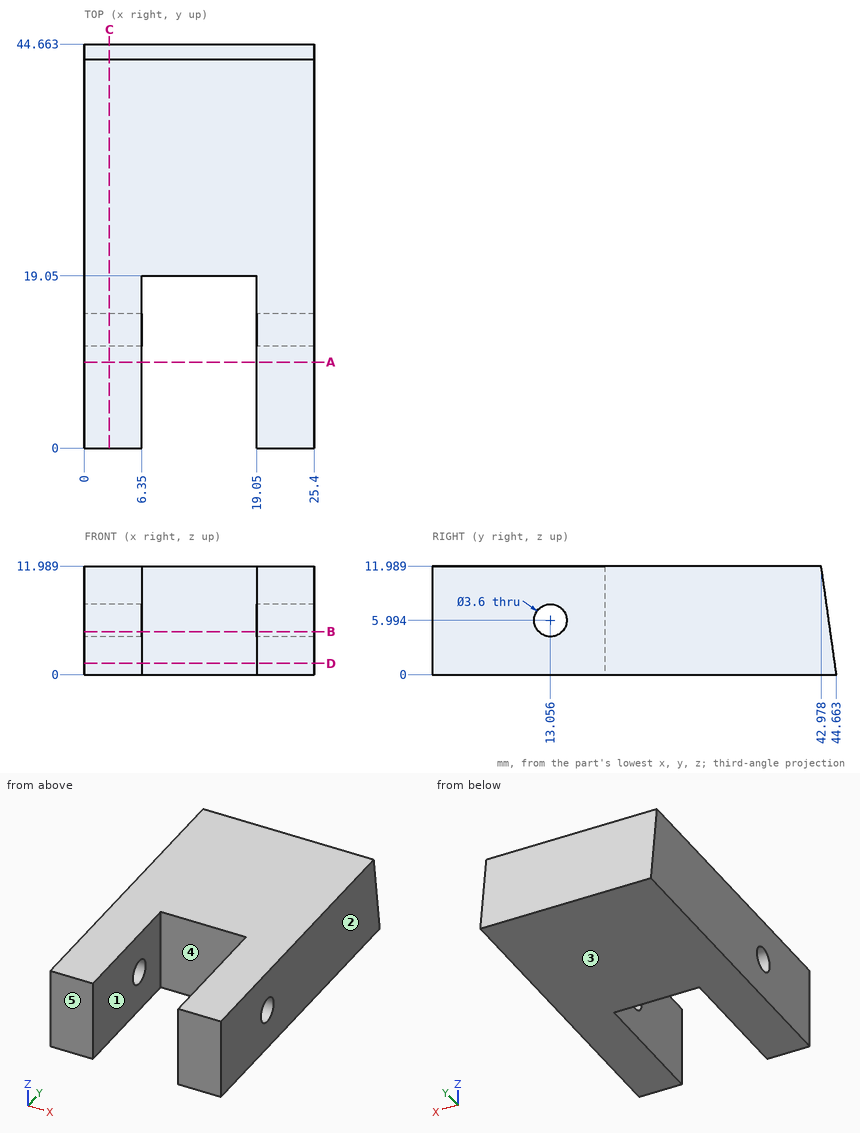
Print and shaded views of the part. All mm, measured from the part's lowest x, y and z. A direction names the side the tool comes from. Give positions to 0.01 mm unless a question says otherwise; leave off trailing zeros. Write each loop counter-clockwise with the first axis right and the second up, starting at its lowest first coordinate (ties: lowest second). Pieces come first, ordered by that corner, then holes. Notation, with made-up numbers: (1.5, 88) - (54.5, 88) arc R27 cw to (54.5, 116) - close; hole circle Ø4 at (44.5, 87.5). An arc over 180 degrees is marked (long way). Put each result on its own line as item: value.
(1) Drop a flat-ended pin along its axis: pin 1 Ø6 at (x, z) = (12, 5.5) entering from -Y. Give the stop position or say it passes through.
Working result:
pin 1: y = 19.05
(2) Wall check: L1, parallel to X at y = 7, z = 11; L2, parallel to Y at x = 23, z = 7.5 (1 decimal); L3, parallel to Z at x = 20, y = 14 (1 decimal). Give the ranges that are in metal, low to high.
Working result:
L1: 0 to 6.35, 19.05 to 25.4
L2: 0 to 12.1, 14 to 43.6
L3: 0 to 4.5, 7.5 to 12
(3) Pull direction X, two halves, no side cores. Call the marked faces 1, 2 and 3: released by +X, released by -X, zero draft, split by the parting line, or undercut.
Working result:
face 1: undercut
face 2: released by +X
face 3: zero draft
(4) Saw through at A-A (y = 9.5). List the corners of the cut face in (x, z), then the cut area to 3 significant figures.
Working result:
outline: (0, 0) - (6.35, 0) - (6.35, 11.99) - (0, 11.99) - close; (19.05, 0) - (25.4, 0) - (25.4, 11.99) - (19.05, 11.99) - close
area: 152 mm^2
(5) Saw through at C-C (x = 2.75). List the corners of the cut face in (y, z) (1 decimal), then the cut area to 3 significant figures.
Working result:
outline: (0, 0) - (44.7, 0) - (43, 12) - (0, 12) - close; hole circle Ø3.6 at (13.1, 6)
area: 515 mm^2
(6) Tool access for the marked faces 4 and 5: list every direction of +Z, -Z, +X, -X, +Y, -Y with a clear straight run to the whole face (end or side of a thin tool).
Working result:
face 4: +Z, -Z, -Y
face 5: +Z, -Z, +X, -X, -Y
(7) Saw through at B-B (z = 4.75). Count the separate pieces of the cut face and the enclosed holes in it.
Working result:
separate pieces: 3
enclosed holes: 0
(8) Saw through at D-D (z = 1.25). List the corners of the cut face in (x, y), then the cut area to 3 significant figures.
Working result:
outline: (0, 0) - (6.35, 0) - (6.35, 19.05) - (19.05, 19.05) - (19.05, 0) - (25.4, 0) - (25.4, 44.49) - (0, 44.49) - close
area: 888 mm^2
